The listing builds one solid part. Answer for the finished solid, in the listing's coordinates (mm). A direction names the side the tool comes from. Give positions to 0.01 mm unless a question says otherwise; leave off trailing zeros. Order: outer loops, then holes, each group sorted by start corner. A loop starts at its lowest first (then second) coordinate and runs counter-clockwise, first axis right, second up. Notation, with made-up numbers: (42.5, -25.5) - (77.5, -25.5) arc R16 ccw to (77.5, 5.5) - close; hole circle Ø6 at (18, 37.5). An arc over 180 degrees is marked (long way). Answer in a Markdown table with one row per item.
from build123d import *

# Parameters (mm, degrees)
SKETCH1_W           = 30.8
SKETCH1_H           = 16.28
BOSS_EXTRUDE1_DEPTH = 28.62
SKETCH3_W           = 5.985
SKETCH3_H           = 2.53
BOSS_EXTRUDE2_DEPTH = 16.28
SKETCH4_W           = 9.61
SKETCH4_H           = 14.41
BOSS_EXTRUDE3_DEPTH = 1
BOSS_EXTRUDE4_DEPTH = 0.73
SKETCH6_R           = 5.52
BOSS_EXTRUDE5_DEPTH = 1.75
CHAMFER1_SIZE       = 1
FILLET1_R           = 1.5
SKETCH7_R           = 1.4
BOSS_EXTRUDE6_DEPTH = 1.47
SKETCH8_R           = 2.48
BOSS_EXTRUDE7_DEPTH = 4
CUT_EXTRUDE1_DEPTH  = 4
SKETCH10_W          = 6.66
SKETCH10_H          = 3.2
BOSS_EXTRUDE8_DEPTH = 1.5
SKETCH11_R          = 0.6
FILLET2_R           = 1.2
FILLET3_R           = 0.6
CHAMFER2_SIZE       = 0.3
SKETCH13_R          = 0.726441042
CUT_EXTRUDE2_DEPTH  = 2.5


with BuildPart() as part:
    # Sketch1 → Boss-Extrude1 (new body)
    with BuildSketch(Plane(origin=(0, 0, 0), x_dir=(1, 0, 0), z_dir=(0, 1, 0))):
        with Locations((15.4, 8.14)):
            Rectangle(SKETCH1_W, SKETCH1_H)
    extrude(amount=BOSS_EXTRUDE1_DEPTH)

    # Sketch3 → Boss-Extrude2 (add)
    with BuildSketch(Plane.XY):
        with Locations((33.7925, 22.775)):
            Rectangle(SKETCH3_W, SKETCH3_H)
        with Locations((-2.9925, 22.775)):
            Rectangle(SKETCH3_W, SKETCH3_H)
    extrude(amount=-BOSS_EXTRUDE2_DEPTH)

    # Sketch4 → Boss-Extrude3 (add)
    with BuildSketch(Plane(origin=(0, 28.62, 0), x_dir=(1, 0, 0), z_dir=(0, 1, 0))):
        with Locations((8.845, 8.14)):
            Rectangle(SKETCH4_W, SKETCH4_H)
    extrude(amount=BOSS_EXTRUDE3_DEPTH)

    # Sketch5 → Boss-Extrude4 (add)
    with BuildSketch(Plane(origin=(0, 28.62, 0), x_dir=(1, 0, 0), z_dir=(0, 1, 0))):
        with BuildLine():
            Line((27.28, 0.985), (16.48, 0.985))
            Line((16.48, 0.985), (16.48, 15.295))
            Line((16.48, 15.295), (27.28, 15.295))
            Line((27.28, 15.295), (27.28, 13.838504907))
            ThreePointArc((27.28, 13.838504907), (30.36, 8.14), (27.28, 2.441495093))
            Line((27.28, 2.441495093), (27.28, 0.985))
        make_face()
    extrude(amount=BOSS_EXTRUDE4_DEPTH)

    # Sketch6 → Boss-Extrude5 (add)
    with BuildSketch(Plane(origin=(0, 29.35, 0), x_dir=(1, 0, 0), z_dir=(0, 1, 0))):
        with Locations((23.07, 8.14)):
            Circle(SKETCH6_R)
    extrude(amount=BOSS_EXTRUDE5_DEPTH)

    # Chamfer1
    chamfer1_edges = [part.edges().sort_by_distance(p)[0] for p in [
        (17.55, 31.1, -8.14),
    ]]
    chamfer(chamfer1_edges, length=CHAMFER1_SIZE)

    # Fillet1
    fillet1_edges = [part.edges().sort_by_distance(p)[0] for p in [
        (27.28, 28.985, -2.441495093),
        (27.28, 28.985, -13.838504907),
    ]]
    fillet(fillet1_edges, radius=FILLET1_R)

    # Sketch7 → Boss-Extrude6 (add)
    with BuildSketch(Plane(origin=(0, 28.62, 0), x_dir=(1, 0, 0), z_dir=(0, 1, 0))):
        with Locations((14.504271984, 8.14)):
            Circle(SKETCH7_R)
    extrude(amount=BOSS_EXTRUDE6_DEPTH)

    # Sketch8 → Boss-Extrude7 (add)
    with BuildSketch(Plane(origin=(0, 31.1, 0), x_dir=(1, 0, 0), z_dir=(0, 1, 0))):
        with Locations((23.07, 8.14)):
            Circle(SKETCH8_R)
    extrude(amount=BOSS_EXTRUDE7_DEPTH)

    # Sketch9 → Cut-Extrude1 (cut)
    with BuildSketch(Plane(origin=(0, 24.04, 0), x_dir=(1, 0, 0), z_dir=(0, 1, 0))):
        with BuildLine():
            Line((37.246499074, 13.14), (37.246499074, 11.14))
            Line((37.246499074, 11.14), (36.132050808, 11.14))
            ThreePointArc((36.132050808, 11.14), (32.4, 12.14), (36.132050808, 13.14))
            Line((36.132050808, 13.14), (37.246499074, 13.14))
        make_face()
        with BuildLine():
            Line((36.132050808, 3.14), (37.246499074, 3.14))
            Line((37.246499074, 3.14), (37.246499074, 5.14))
            Line((37.246499074, 5.14), (36.132050808, 5.14))
            ThreePointArc((36.132050808, 5.14), (32.4, 4.14), (36.132050808, 3.14))
        make_face()
        with BuildLine():
            Line((-5.332050808, 5.14), (-6.446499074, 5.14))
            Line((-6.446499074, 5.14), (-6.446499074, 3.14))
            Line((-6.446499074, 3.14), (-5.332050808, 3.14))
            ThreePointArc((-5.332050808, 3.14), (-1.6, 4.14), (-5.332050808, 5.14))
        make_face()
        with BuildLine():
            Line((-5.332050808, 13.14), (-6.446499074, 13.14))
            Line((-6.446499074, 13.14), (-6.446499074, 11.14))
            Line((-6.446499074, 11.14), (-5.332050808, 11.14))
            ThreePointArc((-5.332050808, 11.14), (-1.6, 12.14), (-5.332050808, 13.14))
        make_face()
    extrude(amount=-CUT_EXTRUDE1_DEPTH, mode=Mode.SUBTRACT)

    # Sketch10 → Boss-Extrude8 (add)
    with BuildSketch(Plane(origin=(30.8, 0, 0), x_dir=(0, 0, -1), z_dir=(1, 0, 0))):
        with Locations((8.14, 9.29)):
            Rectangle(SKETCH10_W, SKETCH10_H)
    extrude(amount=BOSS_EXTRUDE8_DEPTH)

    # Sweep1: sweep along a path in Sketch12
    with BuildLine(Plane(origin=(0, 0, -8.14), x_dir=(-1, 0, 0), z_dir=(0, 0, -1))) as sweep1_path:
        Line((-32.3, 9.27453939), (-33.261270846, 9.27453939))
        ThreePointArc((-33.261270846, 9.27453939), (-38.407623516, 8.601076954), (-43.207388666, 6.626044809))
        Line((-43.207388666, 6.626044809), (-50.146426146, 2.648494581))
    # Sketch11 → Sweep1 (sweep)
    with BuildSketch(Plane(origin=(32.3, 0, 0), x_dir=(0, 0, -1), z_dir=(1, 0, 0))):
        with Locations((6.7940488, 9.27453939)):
            Circle(SKETCH11_R)
        with Locations((8.045254391, 9.27453939)):
            Circle(SKETCH11_R)
        with Locations((9.289971537, 9.27453939)):
            Circle(SKETCH11_R)
    sweep(path=sweep1_path.line)

    # Fillet2
    fillet2_edges = [part.edges().sort_by_distance(p)[0] for p in [
        (-5.985, 22.775, 0),
        (-5.985, 22.775, -16.28),
        (36.785, 22.775, 0),
        (36.785, 22.775, -16.28),
    ]]
    fillet(fillet2_edges, radius=FILLET2_R)

    # Fillet3
    fillet3_edges = [part.edges().sort_by_distance(p)[0] for p in [
        (0, 26.33, 0),
        (0, 10.755, 0),
        (30.8, 10.755, 0),
        (0, 10.755, -16.28),
        (0, 26.33, -16.28),
        (30.8, 26.33, 0),
        (30.8, 26.33, -16.28),
        (30.8, 10.755, -16.28),
    ]]
    fillet(fillet3_edges, radius=FILLET3_R)

    # Chamfer2
    chamfer2_edges = [part.edges().sort_by_distance(p)[0] for p in [
        (20.59, 35.1, -8.14),
    ]]
    chamfer(chamfer2_edges, length=CHAMFER2_SIZE)

    # Sketch13 → Cut-Extrude2 (cut)
    with BuildSketch(Plane(origin=(0, 35.1, 0), x_dir=(1, 0, 0), z_dir=(0, 1, 0))):
        with Locations((23.07, 8.14)):
            Circle(SKETCH13_R)
    extrude(amount=-CUT_EXTRUDE2_DEPTH, mode=Mode.SUBTRACT)


solid = part.part
Item 1: Which of the six approach directions +Z, -Z, +X, -X, +Y, -Y give full straight-line access (tool end or side, diameter ignored) to faces 1 (the face through (32, 9, -11.47)), 2 (the face through (50.14, 2.64, -6.79))?
Answer block:
| item | result |
|---|---|
| face 1 | -Z, +X, -Y |
| face 2 | +Z, -Z, +X, -Y |
Item 2: Each of these flat-tipped pins is pushed along its axis until it touches: P1, Ø0.8, axis at x = 14, z = -8, coming from the +Y side; P2, Ø1.5, axis at x = 20.5, z = -10.5, coming from the +Y side; P3, Ø6.5, axis at x = -3.6, z = -4.14, coming from the -Y side. Where does it stop, or does it pass through?
Answer block:
| item | result |
|---|---|
| P1 | y = 30.09 |
| P2 | y = 31.1 |
| P3 | y = 21.51 |
Item 3: Find section B-B on y = 20. Write down the section's boundary in (x, z).
Answer block:
| item | result |
|---|---|
| outline | (0, -15.68) arc R0.6 ccw to (0.6, -16.28) - (30.2, -16.28) arc R0.6 ccw to (30.8, -15.68) - (30.8, -0.6) arc R0.6 ccw to (30.2, 0) - (0.6, 0) arc R0.6 ccw to (0, -0.6) - close |
Item 4: Consider line 1 (Z direction, x = -3.6, y = 22.6); line 2 (Y direction, x = 32, z = -10.5); line 3 (Z direction, x = 23, y = 33). Determine where each line is inside the solid, lowest interval first.
Answer block:
| item | result |
|---|---|
| line 1 | -16.28 to -14.14, -10.14 to -6.14, -2.14 to 0 |
| line 2 | 7.69 to 10.89, 21.51 to 24.04 |
| line 3 | -10.62 to -8.86, -7.42 to -5.66 |
Item 5: Find section A-A on x = -3.6. Write down the section's boundary in (y, z), then the cut area to 3 significant figures.
Answer block:
| item | result |
|---|---|
| outline | (21.51, -16.28) - (24.04, -16.28) - (24.04, -14.14) - (21.51, -14.14) - close; (21.51, -10.14) - (24.04, -10.14) - (24.04, -6.14) - (21.51, -6.14) - close; (21.51, -2.14) - (24.04, -2.14) - (24.04, 0) - (21.51, 0) - close |
| area | 20.9 mm² |
Item 6: Find section D-D on x = 34.4. Count the separate pieces of the cut face and the enclosed holes in it, then the cut area to 3 significant figures.
Answer block:
| item | result |
|---|---|
| separate pieces | 6 |
| enclosed holes | 0 |
| area | 24.3 mm² |
Item 7: Determine the mould class of faces 3 (the face through (46.977, 5.048, -7.117)), 4 (the face through (32.79, 8.74, -7.07)), 5 (the face through (24, 35.1, -8)), 6 (the face through (21.242, 32.924, -9.816)) for opening direction X: pulls with the +X half, pulls with the -X half, needs draft (parallel to the pull), parting line crosses it, or undercut.
Answer block:
| item | result |
|---|---|
| face 3 | undercut |
| face 4 | undercut |
| face 5 | needs draft |
| face 6 | parting line crosses it |
Item 8: Find section C-C on x = 23.07. Write down the section's boundary in (y, z) (3 decimals), then the cut area to 3 significant figures.
Answer block:
| item | result |
|---|---|
| outline | (0, -16.28) - (28.62, -16.28) - (28.62, -15.295) - (29.35, -15.295) - (29.35, -13.66) - (30.1, -13.66) - (31.1, -12.66) - (31.1, -10.62) - (34.8, -10.62) - (35.1, -10.32) - (35.1, -8.866) - (32.6, -8.866) - (32.6, -7.414) - (35.1, -7.414) - (35.1, -5.96) - (34.8, -5.66) - (31.1, -5.66) - (31.1, -3.62) - (30.1, -2.62) - (29.35, -2.62) - (29.35, -0.985) - (28.62, -0.985) - (28.62, 0) - (0, 0) - close |
| area | 511 mm² |
